Can you work these out from the model? Positions are in its coordinate system, mm. A direction names the side the tool comes from. Round coordinates to 2 decimals unless told otherwise and drop trailing zeros. Loops run counter-clockwise (first coordinate to the right, second up) from the corner with the lowest first, then second, coordinate; pieces in that order, holes last. Notation, with made-up numbers: (-31, -22) -> (-6, -22) arc R25 ccw to (-6, -5) -> close; hole circle Ø4 at (21.25, 8.25). An arc over 180 degrees is marked (long way). Use a Markdown table: item, result.
from build123d import *

# Parameters (mm, degrees)
CROQUIS1_R              = 1.25
CROQUIS1_R_2            = 1.5
CROQUIS1_R_3            = 16.75
CROQUIS1_R_4            = 1.1
SALIENTE_EXTRUIR1_DEPTH = 1.6


with BuildPart() as part:
    # Croquis1 → Saliente-Extruir1 (new body)
    with BuildSketch(Plane(origin=(0, 0, 0), x_dir=(1, 0, 0), z_dir=(0, 1, 0))):
        Polygon((65.571001722, 3.859007926), (61.644001722, 3.859007926), (59.104001722, 1.975007926), (54.333001722, -0.155992074), (33.470001722, -0.155992074), (29.893001722, 4.670007926), (12.949494381, 4.670007926), (9.375001722, 7.926e-06), (1.722e-06, 7.926e-06), (1.722e-06, 2.277007926), (0.872001722, 3.207007926), (0.872001722, 21.491007926), (0.872001722, 33.587260304), (-1.536998278, 34.539963538), (-1.536998278, 49.146007926), (-6.824998278, 52.811007926), (-6.824998278, 56.199007926), (-4.886998278, 57.460007926), (-4.886998278, 66.704007926), (-6.153998278, 68.325007926), (-6.153998278, 76.772007926), (-2.987377359, 76.772007926), (12.949494381, 76.772007926), (36.470001722, 81.705007926), (90.745001722, 81.705007926), (114.265509063, 76.772007926), (130.202380802, 76.772007926), (133.369001722, 76.772007926), (133.369001722, 68.325007926), (132.102001722, 66.704007926), (132.102001722, 57.460007926), (134.040001722, 56.199007926), (134.040001722, 52.811007926), (128.752001722, 49.146007926), (128.752001722, 34.539963538), (126.343001722, 33.587260304), (126.343001722, 21.491007926), (126.343001722, 3.207007926), (127.215001722, 2.277007926), (127.215001722, 7.926e-06), (117.840001722, 7.926e-06), (114.265509063, 4.670007926), (97.322001722, 4.670007926), (93.745001722, -0.155992074), (72.882001722, -0.155992074), (68.111001722, 1.975007926), align=None)
        with Locations(Location((5.998001722, 11.001007926, 0), (0, 0, 270))):
            Circle(CROQUIS1_R, mode=Mode.SUBTRACT)
        with Locations(Location((5.998001722, 36.001007926, 0), (0, 0, 270))):
            Circle(CROQUIS1_R, mode=Mode.SUBTRACT)
        with Locations(Location((121.217001722, 36.001007926, 0), (0, 0, 270))):
            Circle(CROQUIS1_R, mode=Mode.SUBTRACT)
        with Locations(Location((121.217001722, 11.001007926, 0), (0, 0, 270))):
            Circle(CROQUIS1_R, mode=Mode.SUBTRACT)
        with Locations(Location((-0.950998278, 71.841007926, 0), (0, 0, 270))):
            Circle(CROQUIS1_R_2, mode=Mode.SUBTRACT)
        with Locations(Location((-0.950998278, 64.841007926, 0), (0, 0, 270))):
            Circle(CROQUIS1_R_2, mode=Mode.SUBTRACT)
        with Locations(Location((17.167001722, 71.285007926, 0), (0, 0, 270))):
            Circle(CROQUIS1_R, mode=Mode.SUBTRACT)
        with Locations(Location((54.929001722, 79.176007926, 0), (0, 0, 270))):
            Circle(CROQUIS1_R, mode=Mode.SUBTRACT)
        with Locations(Location((29.998001722, 36.001007926, 0), (0, 0, 270))):
            Circle(CROQUIS1_R, mode=Mode.SUBTRACT)
        with Locations(Location((29.998001722, 11.001007926, 0), (0, 0, 270))):
            Circle(CROQUIS1_R, mode=Mode.SUBTRACT)
        with Locations(Location((97.217001722, 11.001007926, 0), (0, 0, 270))):
            Circle(CROQUIS1_R, mode=Mode.SUBTRACT)
        with Locations(Location((97.217001722, 36.001007926, 0), (0, 0, 270))):
            Circle(CROQUIS1_R, mode=Mode.SUBTRACT)
        with Locations(Location((72.286001722, 79.176007926, 0), (0, 0, 270))):
            Circle(CROQUIS1_R, mode=Mode.SUBTRACT)
        with Locations(Location((110.048001722, 71.285007926, 0), (0, 0, 270))):
            Circle(CROQUIS1_R, mode=Mode.SUBTRACT)
        with Locations(Location((128.166001722, 64.841007926, 0), (0, 0, 270))):
            Circle(CROQUIS1_R_2, mode=Mode.SUBTRACT)
        with Locations(Location((128.166001722, 71.841007926, 0), (0, 0, 270))):
            Circle(CROQUIS1_R_2, mode=Mode.SUBTRACT)
        with Locations(Location((63.607501722, 27.859007926, 0), (0, 0, 270))):
            Circle(CROQUIS1_R_3, mode=Mode.SUBTRACT)
        with Locations(Location((63.607501722, 48.779312854, 0), (0, 0, 270))):
            Circle(CROQUIS1_R_4, mode=Mode.SUBTRACT)
        with Locations(Location((84.52780665, 27.859007926, 0), (0, 0, 270))):
            Circle(CROQUIS1_R_4, mode=Mode.SUBTRACT)
        with Locations(Location((63.607501722, 6.938702998, 0), (0, 0, 270))):
            Circle(CROQUIS1_R_4, mode=Mode.SUBTRACT)
        with Locations(Location((42.687196794, 27.859007926, 0), (0, 0, 270))):
            Circle(CROQUIS1_R_4, mode=Mode.SUBTRACT)
    extrude(amount=SALIENTE_EXTRUIR1_DEPTH)


solid = part.part
1. Which directions (+Z, -Z, +X, -X, +Y, -Y) give clear straight access to the entire face, cutting with the end or side of a thin tool? Please do faces 4 (the cylindrical face through (6.05, 0.79, -37.25)), 5 (the flat face through (95.56, 0.79, -2.29)).
Answer sheet:
| item | result |
|---|---|
| face 4 | +Y, -Y |
| face 5 | +Z, +Y, -Y |
2. I want a section at B-B (x = 78). Please give me the cut outline in (y, z) (3 decimals), plus the area to 3 significant figures.
Answer sheet:
| item | result |
|---|---|
| outline | (0, -81.705) -> (1.6, -81.705) -> (1.6, -36.427) -> (0, -36.427) -> close; (0, -19.291) -> (1.6, -19.291) -> (1.6, 0.156) -> (0, 0.156) -> close |
| area | 104 mm² |
3. I want a section at A-A (z = -20.5). Please give me the cut outline in (x, y).
Answer sheet:
| item | result |
|---|---|
| outline | (0.87, 0) -> (48.56, 0) -> (48.56, 1.6) -> (0.87, 1.6) -> close; (78.65, 0) -> (126.34, 0) -> (126.34, 1.6) -> (78.65, 1.6) -> close |
4. I want a section at C-C (y = 1). State how many separate pieces and enclosed holes the cut face has, plus the area to 3 significant figures.
Answer sheet:
| item | result |
|---|---|
| separate pieces | 1 |
| enclosed holes | 21 |
| area | 9,240 mm² |
5. Will these pins go through, and if not, where does the flat tip stop? pin 1 Ø4 at (x, z) = (97.22, -36) entering from +Y; pin 2 Ø0.5 at (y, z) = (0.5, -39) entering from -X; pin 3 Ø0.8 at (y, z) = (0.5, -25.5) entering from -X; pin 4 Ø0.8 at (x, y) = (17.5, 1) entering from +Z.
Answer sheet:
| item | result |
|---|---|
| pin 1 | stops at y = 1.6 |
| pin 2 | stops at x = -1.54 |
| pin 3 | stops at x = 0.87 |
| pin 4 | stops at z = -4.67 |
6. I need wall thicknesses on line 1 (X direction, y = 1.15, z = -28); line 2 (Z direction, x = 72, y = 0.85) (3 decimals); line 3 (X direction, y = 1, z = -7). Which ranges of each line are inside material? Lowest first, please.
Answer sheet:
| item | result |
|---|---|
| line 1 | x = 0.87 to 41.6, 43.78 to 46.86, 80.36 to 83.44, 85.62 to 126.34 |
| line 2 | z = -81.705 to -80.393, -77.959 to -42.355, -13.363 to -0.238 |
| line 3 | x = 0.87 to 62.51, 64.71 to 126.34 |
7. If we mould it in two halves opening along X, with no side actions, what happens to faces 1 (the flat face through (116.08, 0.79, -2.3)), 2 (the flat face through (24.545, 0.789, -79.204)), 3 (the flat face through (65, 0, -50))? For each: +X half, -X half, draft (parallel to the pull), parting line (faces both ways), or undercut.
Answer sheet:
| item | result |
|---|---|
| face 1 | undercut |
| face 2 | -X half |
| face 3 | draft |
8. I want a section at D-D (x = 102). Please give me the cut outline in (y, z), plus the area to 3 significant figures.
Answer sheet:
| item | result |
|---|---|
| outline | (0, -79.34) -> (1.6, -79.34) -> (1.6, -4.67) -> (0, -4.67) -> close |
| area | 119 mm² |
